The model under review builds one solid part; all positions refer to its coordinate system, in mm. Face numbers are marked on the shaded views. A direction names the side the tool comes from. Coordinates: 2 decimals unless noted, no trailing zeros. Write each loop counter-clockwise with the first axis right and the second up, starting at its lowest first coordinate (ties: lowest second). Pieces come first, ordered by that corner, then holes. Notation, with made-up numbers: (79.5, -10) - (111.5, -10) arc R26 cw to (111.5, 9) - close; hole circle Ø4 at (48.25, 59.5). An arc over 180 degrees is marked (long way). Put each result on its own line as item: value.
from build123d import *

# Parameters (mm, degrees)
SKETCH1_R           = 18.75
BOSS_EXTRUDE1_DEPTH = 50
SKETCH2_R           = 6.55
BOSS_EXTRUDE2_DEPTH = 5
SKETCH3_R           = 1.6
BOSS_EXTRUDE3_DEPTH = 8
SKETCH4_R           = 6.5
BOSS_EXTRUDE4_DEPTH = 2.5
SKETCH5_R           = 4
BOSS_EXTRUDE5_DEPTH = 1.3
SKETCH6_W           = 0.5
SKETCH6_H           = 3.85
BOSS_EXTRUDE6_DEPTH = 7


with BuildPart() as part:
    # Sketch1 → Boss-Extrude1 (new body)
    with BuildSketch(Plane(origin=(0, 0, 0), x_dir=(1, 0, 0), z_dir=(0, 1, 0))):
        with Locations(Location((0, 0, 0), (0, 0, 270))):
            Circle(SKETCH1_R)
    extrude(amount=BOSS_EXTRUDE1_DEPTH)

    # Sketch2 → Boss-Extrude2 (add)
    with BuildSketch(Plane(origin=(0, 50, 0), x_dir=(1, 0, 0), z_dir=(0, 1, 0))):
        with Locations(Location((0, 0, 0), (0, 0, 270))):
            Circle(SKETCH2_R)
    extrude(amount=BOSS_EXTRUDE2_DEPTH)

    # Sketch3 → Boss-Extrude3 (add)
    with BuildSketch(Plane(origin=(0, 55, 0), x_dir=(1, 0, 0), z_dir=(0, 1, 0))):
        with Locations(Location((0, 0, 0), (0, 0, 270))):
            Circle(SKETCH3_R)
    extrude(amount=BOSS_EXTRUDE3_DEPTH)

    # Sketch4 → Boss-Extrude4 (add)
    with BuildSketch(Plane.XZ):
        with Locations(Location((0, 0, 0), (0, 0, 90))):
            Circle(SKETCH4_R)
    extrude(amount=BOSS_EXTRUDE4_DEPTH)

    # Sketch5 → Boss-Extrude5 (add)
    with BuildSketch(Plane.XZ.offset(2.5)):
        with Locations(Location((0, 0, 0), (0, 0, 270))):
            Circle(SKETCH5_R)
    extrude(amount=BOSS_EXTRUDE5_DEPTH)

    # Sketch6 → Boss-Extrude6 (add)
    with BuildSketch(Plane.XZ):
        with Locations((-14, 0)):
            Rectangle(SKETCH6_W, SKETCH6_H)
        with Locations((14, 0)):
            Rectangle(SKETCH6_W, SKETCH6_H)
    extrude(amount=BOSS_EXTRUDE6_DEPTH)


solid = part.part
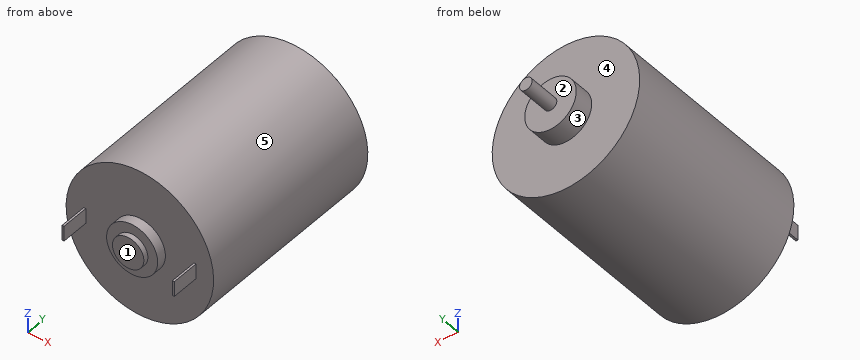
1. For pin 1 Ø4 at (x, z) = (2.5, -0.5) entering from -Y; pin 2 Ø4 at (y, z) = (11.5, -9) entering from -X; pin 3 Ø4 at (x, z) = (-14, 6) entering from -Y, all flat-tipped, find the tip position at first contact; note any pin that passes through.
Determined:
pin 1: stops at y = -3.8
pin 2: stops at x = -17.39
pin 3: stops at y = 0
2. Consider section C-C on y = 9.5. State the section outline as (x, z) points.
Determined:
outline: circle Ø37.5 at (0, 0)
3. Consider section D-D on z = 15. State the section outline as (x, y) points, plus the area to 4 significant figures.
Determined:
outline: (-11.25, 0) - (11.25, 0) - (11.25, 50) - (-11.25, 50) - close
area: 1,125 mm^2
4. To check wall thickness, follow probe 1 along Y at (x, z) = (-8.5, 9.5); probe 2 along X at (y, z) = (29, 0.5); probe 3 along Z at (x, y) = (-6.5, 10.5). State the ranges of each line that lie inside material, in increasing order.
Determined:
probe 1: y = 0 to 50
probe 2: x = -18.74 to 18.74
probe 3: z = -17.59 to 17.59
5. Machinability: for the marked faces 4 and 5, which of the approach directions +Z, -Z, +X, -X, +Y, -Y give a long, thin tool a straight path to every point of the face, cutting with its end or side? Answer none if there is none.
Determined:
face 4: +Y
face 5: +Y, -Y
6. Consider section A-A on x = 0. State the section outline as (y, z) points.
Determined:
outline: (-3.8, -4) - (-2.5, -4) - (-2.5, -6.5) - (0, -6.5) - (0, -18.75) - (50, -18.75) - (50, -6.55) - (55, -6.55) - (55, -1.6) - (63, -1.6) - (63, 1.6) - (55, 1.6) - (55, 6.55) - (50, 6.55) - (50, 18.75) - (0, 18.75) - (0, 6.5) - (-2.5, 6.5) - (-2.5, 4) - (-3.8, 4) - close
7. Consider section B-B on z = 0. State the section outline as (x, y) points.
Determined:
outline: (-18.75, 0) - (-14.25, 0) - (-14.25, -7) - (-13.75, -7) - (-13.75, 0) - (-6.5, 0) - (-6.5, -2.5) - (-4, -2.5) - (-4, -3.8) - (4, -3.8) - (4, -2.5) - (6.5, -2.5) - (6.5, 0) - (13.75, 0) - (13.75, -7) - (14.25, -7) - (14.25, 0) - (18.75, 0) - (18.75, 50) - (6.55, 50) - (6.55, 55) - (1.6, 55) - (1.6, 63) - (-1.6, 63) - (-1.6, 55) - (-6.55, 55) - (-6.55, 50) - (-18.75, 50) - close
8. The part is to be moulded in two halves that separate along X. For the marked faces 1, 2 and 3, say which applies: +X half, -X half, draft (parallel to the pull), parting line (faces both ways), or undercut.
Determined:
face 1: undercut
face 2: draft
face 3: parting line
